Part model, mm, in its own coordinate system. A direction names the side the tool comes from. Round coordinates to 2 decimals unless told otherwise and drop trailing zeros. Write each loop counter-clockwise with the first axis right and the second up, starting at its lowest first coordinate (ties: lowest second). Pieces come first, ordered by that corner, then holes. Notation, with made-up numbers: M 62,80.25 L 113,80.25 A4 cw 113,86.25 Z; hole C -21.5,3.25 d5. An arc over 180 degrees is marked long. Use one line per item in the form item = value. Start each with the question number.
Item 1: Cut at C-C, the plane y = -13.75. Give the cut face in (x, z), then the cut area to 3 significant figures.
Item 2: Which spindle directions (+Z, -Z, +X, -X, +Y, -Y) get a long thin tool onto all of the face, cutting with end or side? Do faces 5 (the face through (27.9, -2.58, -0.36)), 6 (the face through (0.356, -23.872, -23.951)), 7 (the face through (0, -13, -22.86)). Say none if no direction does.
Item 3: Cut at D-D, the plane x = 19. Give the cut face in (y, z), then the cut area to 3 significant figures.
Item 4: Cut at A-A, the plane y = -3.75. Give the cut face in (x, z).
Item 5: Probe L1, parallel to X at y = -14.25, z = -7; L2, parallel to Z at x = 42.5, y = -13.75; L3, parallel to X at y = -5.25, z = -3.5. List the from-to ranges inside material, lowest first.
Item 6: Flat gauge pins, fed straight in: pin 1 Ø1.5 at (x, y) = (-6, -21.5) entering from +Z; pin 2 Ø2 at (x, y) = (49.5, -4) entering from +Z; pin 3 Ø1.5 at (x, z) = (54, -1) entering from +Y. Where does each tip first touch, or does it go through?
Item 7: Mould opens along X. For faces 1 (the face through (28.664, -22.096, 0.32)), 2 (the face through (70.55, -3.02, -0.32)), 3 (the face through (0.356, -23.872, 23.951)), 4 (the face through (-22.82, -2.5, -0.36)) say: +X half, -X half, draft (parallel to the pull), parting line (faces both ways), or undercut.
from build123d import *

# Parameters (mm, degrees)
F0_W     = 50.8
F0_H     = 50.8
F1_DEPTH = 25.4
F3_R     = 5.08
F4_SIZE  = 5.08
F5_T     = -2.54


# Not quite as in the source:
# - a feature of the source that left no trace in its solid (it failed there, or was rolled back) is left out


with BuildPart() as f1:
    # F0 (on Front) → F1 (new body)
    with BuildSketch(Plane.XZ):
        Rectangle(F0_W, F0_H)
    extrude(amount=F1_DEPTH)

    # F3
    f3_edges = [f1.edges().sort_by_distance(p)[0] for p in [
        (0, -25.4, 25.4),
        (-25.4, -25.4, 0),
        (0, -25.4, -25.4),
        (25.4, -25.4, 0),
    ]]
    fillet(f3_edges, radius=F3_R)

    # F4
    f4_edges = [f1.edges().sort_by_distance(p)[0] for p in [
        (0, 0, 25.4),
        (-25.4, 0, 0),
        (0, 0, -25.4),
        (25.4, 0, 0),
    ]]
    chamfer(f4_edges, length=F4_SIZE)

    # F5
    f5_openings = [f1.faces().sort_by_distance(p)[0] for p in [
        (0, 0, 0),
    ]]
    offset(amount=F5_T, openings=f5_openings)

    # F6: F1 across face


with BuildPart() as f1_1:
    add(f1.part)
    add(f1.part.mirror(Plane(origin=(25.4, -12.7, 0), x_dir=(0, 1, 0), z_dir=(1, 0, 0))))


solid = f1_1.part
Model answer:
q1.outline = M -25.4,-25.4 L 76.2,-25.4 L 76.2,25.4 L -25.4,25.4 Z; hole M -22.86,-22.86 L 22.86,-22.86 L 22.86,22.86 L -22.86,22.86 Z; hole M 27.94,-22.86 L 73.66,-22.86 L 73.66,22.86 L 27.94,22.86 Z
q1.area = 981 mm²
q2.face_5 = +Z, -Z, +Y
q2.face_6 = -Z, +X, -X, -Y
q2.face_7 = none
q3.outline = M -25.4,-20.32 A5.08 ccw -20.32,-25.4 L -5.08,-25.4 L 0,-20.32 L 0,20.32 L -5.08,25.4 L -20.32,25.4 A5.08 ccw -25.4,20.32 Z; hole M -22.86,-20.32 A2.54 ccw -20.32,-22.86 L -6.13,-22.86 L -2.27,-19 L -2.27,19 L -6.13,22.86 L -20.32,22.86 A2.54 ccw -22.86,20.32 Z
q3.area = 330 mm²
q4.outline = M -24.07,-24.07 L 24.07,-24.07 L 24.07,24.07 L -24.07,24.07 Z; M 26.73,-24.07 L 74.87,-24.07 L 74.87,24.07 L 26.73,24.07 Z; hole M -20.48,-20.48 L 20.48,-20.48 L 20.48,20.48 L -20.48,20.48 Z; hole M 30.32,-20.48 L 71.28,-20.48 L 71.28,20.48 L 30.32,20.48 Z
q5.L1 = -25.4 to -22.86, 22.86 to 27.94, 73.66 to 76.2
q5.L2 = -25.4 to -22.86, 22.86 to 25.4
q5.L3 = -25.4 to -21.98, 21.98 to 28.82, 72.78 to 76.2
q6.pin_1 = 25.38
q6.pin_2 = 25.32
q6.pin_3 = -22.86
q7.face_1 = undercut
q7.face_2 = undercut
q7.face_3 = draft
q7.face_4 = -X half
